```python
from build123d import *

# Parameters (mm, degrees)
SKETCH_1_R               = 16.85
EXTRUDE_1_DEPTH          = 12
FILLET_1_R               = 30
FILLET_2_R               = 60
CUT_EXTRUDE_1_DEPTH      = 410.990466147
CUT_EXTRUDE_1_DEPTH_BACK = 410.990466147
FILLET_3_R               = 2
FILLET_4_R               = 20
CUT_EXTRUDE_2_DEPTH      = 410.868383554
CUT_EXTRUDE_2_DEPTH_BACK = 410.868383554
EXTRUDE_START            = -12
EXTRUDE_2_DEPTH          = 12


with BuildPart() as part:
    # Sketch 1 → Бобышка-Вытянуть1 (new body)
    with BuildSketch(Plane.XY):
        with BuildLine():
            Line((-1.020104874, -24.979179051), (115.882453083, -29.75326986))
            Line((115.882453083, -29.75326986), (121.310616212, -114.579769523))
            Line((121.310616212, -114.579769523), (108.583485608, -371.264440173))
            Line((108.583485608, -371.264440173), (128.558946359, -372.254878352))
            Line((128.558946359, -372.254878352), (171.389870978, -114.220142814))
            Line((171.389870978, -114.220142814), (162.905370512, 18.368075133))
            Line((162.905370512, 18.368075133), (1.020104874, 24.979179051))
            ThreePointArc((1.020104874, 24.979179051), (-24.979179051, 1.020104874), (-1.020104874, -24.979179051))
        make_face()
        Circle(SKETCH_1_R, mode=Mode.SUBTRACT)
    extrude(amount=EXTRUDE_1_DEPTH)

    # Скругление1
    fillet_1_edges = [part.edges().sort_by_distance(p)[0] for p in [
        (115.882453083, -29.75326986, 6),
    ]]
    fillet(fillet_1_edges, radius=FILLET_1_R)

    # Скругление2
    fillet_2_edges = [part.edges().sort_by_distance(p)[0] for p in [
        (162.905370512, 18.368075133, 6),
    ]]
    fillet(fillet_2_edges, radius=FILLET_2_R)

    # Sketch 2 → Вырез-Вытянуть1 (cut, two sides: drawn at the far end of the back side and taken through both)
    with BuildSketch(Plane(origin=(0, 0, 0), x_dir=(-1, 0, 0), z_dir=(0, 0, -1)).offset(-CUT_EXTRUDE_1_DEPTH_BACK)):
        Polygon((-108.583485608, -371.264440173), (-116.573669908, -371.660615445), (-118.40598054, -334.706013056), (-110.41579624, -334.309837784), align=None)
    extrude(amount=CUT_EXTRUDE_1_DEPTH + CUT_EXTRUDE_1_DEPTH_BACK, mode=Mode.SUBTRACT)

    # Скругление3
    fillet_3_edges = [part.edges().sort_by_distance(p)[0] for p in [
        (128.558946359, -372.254878352, 6),
    ]]
    fillet(fillet_3_edges, radius=FILLET_3_R)

    # Скругление4
    fillet_4_edges = [part.edges().sort_by_distance(p)[0] for p in [
        (171.389870978, -114.220142814, 6),
    ]]
    fillet(fillet_4_edges, radius=FILLET_4_R)

    # Эскиз3 → Вырез-Вытянуть2 (cut, two sides: drawn at the far end of the back side and taken through both)
    with BuildSketch(Plane.XY.offset(12).offset(-CUT_EXTRUDE_2_DEPTH_BACK)):
        with BuildLine():
            Line((13.955291323, -25.590747374), (88.892828475, -28.651061996))
            ThreePointArc((88.892828475, -28.651061996), (108.635605286, -37.16939974), (117.607467213, -56.710254576))
            Line((117.607467213, -56.710254576), (121.310616212, -114.579769523))
            Line((121.310616212, -114.579769523), (110.41579624, -334.309837784))
            Line((110.41579624, -334.309837784), (113.412115352, -334.458403511))
            Line((113.412115352, -334.458403511), (124.315371498, -114.558191921))
            Line((124.315371498, -114.558191921), (120.601343672, -56.518672348))
            ThreePointArc((120.601343672, -56.518672348), (110.732295552, -35.023732029), (89.01524106, -25.65356051))
            Line((89.01524106, -25.65356051), (13.955291323, -22.588246777))
            Line((13.955291323, -22.588246777), (13.955291323, -25.590747374))
        make_face()
    extrude(amount=CUT_EXTRUDE_2_DEPTH + CUT_EXTRUDE_2_DEPTH_BACK, mode=Mode.SUBTRACT)

    # Эскиз4 → Бобышка-Вытянуть2 (add)
    with BuildSketch(Plane.XY.offset(12).offset(EXTRUDE_START)):
        with BuildLine():
            Line((120.601343672, -56.518672348), (119.104405442, -56.614463462))
            ThreePointArc((119.104405442, -56.614463462), (109.683950419, -36.096565885), (88.954034767, -27.152311253))
            Line((88.954034767, -27.152311253), (89.01524106, -25.65356051))
            ThreePointArc((89.01524106, -25.65356051), (110.732295552, -35.023732029), (120.601343672, -56.518672348))
        make_face()
    extrude(amount=EXTRUDE_2_DEPTH)


solid = part.part
```
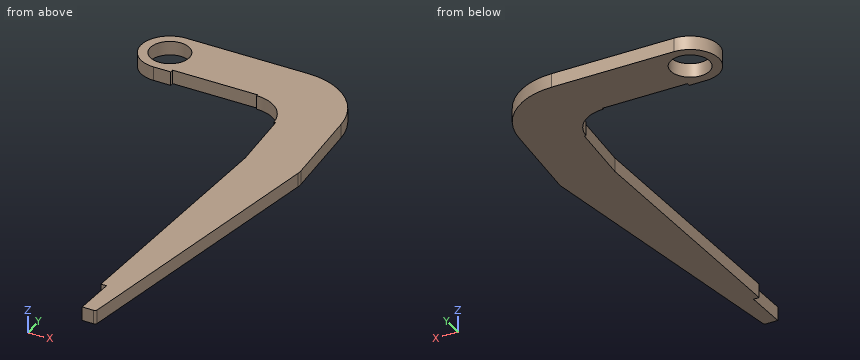
Check sheet for the modelled part. Datum: model origin and axes. Units: mm. Round coordinates to 2 decimals unless told otherwise and drop trailing zeros. Order: outer loops, then holes, each group sorted by start corner. A loop starts at its lowest first (then second) coordinate and runs counter-clockwise, first axis right, second up. Notation, with made-up numbers: (47.25, 88) -> (81.25, 88) arc R25 ccw to (81.25, 127) -> close; hole circle Ø3 at (61, 59.25). An arc over 180 degrees is marked (long way). One line per item, written item: value. Start each with the question number.
Q1. Cross-section at A-A (z = 3). Record the boundary of the cut face in (x, y), and give its area (3 significant figures).
Q2. Cross-section at D-D (y = -103). Record the boundary of the cut face in (x, z).
Q3. Thickness scan on line 1 (Y direction, x = 0, z = 9.25); line 2 (X direction, y = 7, z = 4); line 3 (X direction, y = -272.5, z = 7.5). Record the ranges inside material, lowest first.
Q4. Cross-section at C-C (x = 77.5). Record the boundary of the cut face in (y, z).
Q5. Gauge pin test, flat ends, axial feed: pin 1 Ø3.5 at (y, z) = (-23.5, 7.5) entering from +X; pin 2 Ø6 at (y, z) = (-301, 5.5) entering from -X; pin 3 Ø3 at (x, z) = (37, 3.5) entering from -Y. Record the tip position at first contact, or that the pin passes through.
Q6. Cross-section at B-B (y = 0). Record the boundary of the cut face in (x, z).
Completed:
1. outline: (-1.02, -24.98) -> (13.96, -25.59) -> (13.96, -22.59) -> (89.02, -25.65) -> (88.95, -27.15) arc R31.5 cw to (119.1, -56.61) -> (120.6, -56.52) -> (124.32, -114.56) -> (113.41, -334.46) -> (118.41, -334.71) -> (116.57, -371.66) -> (126.78, -372.17) arc R2 ccw to (128.85, -370.5) -> (171.01, -116.48) arc R20 ccw to (171.24, -111.93) -> (166.36, -35.55) arc R60 ccw to (108.93, 20.57) -> (1.02, 24.98) arc R25 ccw to start; hole circle Ø33.7 at (0, 0)
1. area: 19,700 mm²
2. outline: (123.58, 0) -> (170.67, 0) -> (170.67, 12) -> (123.58, 12) -> close
3. line 1: y = -25.02 to -16.85, 16.85 to 25
3. line 2: x = -24 to -15.33, 15.33 to 144.55
3. line 3: x = 116.48 to 145.12
4. outline: (-25.18, 0) -> (21.86, 0) -> (21.86, 12) -> (-25.18, 12) -> close
5. pin 1: stops at x = 164.79
5. pin 2: stops at x = 114.92
5. pin 3: stops at y = -23.59
6. outline: (-25, 0) -> (-16.85, 0) -> (-16.85, 12) -> (-25, 12) -> close; (16.85, 0) -> (151.75, 0) -> (151.75, 12) -> (16.85, 12) -> close
